```python
from build123d import *

# Parameters (mm, degrees)
EXTRU_MINCE1_DEPTH         = 2.3
CONG_1_R                   = 2.3
ESQUISSE2_W                = 40
ESQUISSE2_H                = 49.6
BOSS_EXTRU_1_DEPTH         = 2.3
R_P_TITION_LIN_AIRE1_COUNT = 2
R_P_TITION_LIN_AIRE1_PITCH = 40
CONG_2_R                   = 2.3
BOSS_EXTRU_2_DEPTH         = 40
ENL_V_START                = 37.8
ESQUISSE4_W                = 30
ESQUISSE4_H                = 12
ENL_V_MAT_EXTRU_1_DEPTH    = 35.5


with BuildPart() as part:
    # Esquisse1 → Extru.-Mince1 (new, symmetric)
    with BuildSketch(Plane.XY):
        Polygon((-4.3, -57), (-4.3, -47.3), (2.3, -47.3), (2.3, 2.3), (-8.9, 2.3), (-8.9, -12), (-4.3, -12), (-4.3, -2.3), (-2.3, -2.3), (-2.3, -42.7), (-8.9, -42.7), (-8.9, -57), align=None)
    extru_mince1 = extrude(amount=EXTRU_MINCE1_DEPTH, both=True)

    # Congé1
    cong_1_edges = [part.edges().sort_by_distance(p)[0] for p in [
        (-6.6, -57, -2.3),
        (-4.3, -52.15, -2.3),
        (-1, -47.3, -2.3),
        (2.3, -22.5, -2.3),
        (-3.3, 2.3, -2.3),
        (-8.9, -4.85, -2.3),
        (-6.6, -12, -2.3),
        (-4.3, -7.15, -2.3),
        (-3.3, -2.3, -2.3),
        (-2.3, -22.5, -2.3),
        (-5.6, -42.7, -2.3),
        (-8.9, -49.85, -2.3),
        (-5.6, -42.7, 2.3),
        (-2.3, -22.5, 2.3),
        (-3.3, -2.3, 2.3),
        (-4.3, -7.15, 2.3),
        (-6.6, -12, 2.3),
        (-8.9, -4.85, 2.3),
        (-3.3, 2.3, 2.3),
        (2.3, -22.5, 2.3),
        (-1, -47.3, 2.3),
        (-4.3, -52.15, 2.3),
        (-6.6, -57, 2.3),
        (-8.9, -49.85, 2.3),
    ]]
    fillet(cong_1_edges, radius=CONG_1_R - 0.0001)  # a hair under: the kernel refuses the full size

    # Esquisse2 → Boss.-Extru.1 (add)
    with BuildSketch(Plane(origin=(0, 0, 0), x_dir=(0, 0, -1), z_dir=(1, 0, 0))):
        with Locations((-20, -22.5)):
            Rectangle(ESQUISSE2_W, ESQUISSE2_H)
    extrude(amount=BOSS_EXTRU_1_DEPTH)

    # Répétition linéaire1: Extru.-Mince1 ×2
    with Locations(*[(0, 0, i * R_P_TITION_LIN_AIRE1_PITCH) for i in range(1, R_P_TITION_LIN_AIRE1_COUNT)]):
        add(extru_mince1)

    # Congé2
    cong_2_edges = [part.edges().sort_by_distance(p)[0] for p in [
        (-5.6, -42.7, 42.3),
        (-2.3, -22.5, 42.3),
        (-3.3, -2.3, 42.3),
        (-4.3, -7.15, 42.3),
        (-6.6, -12, 42.3),
        (-8.9, -4.85, 42.3),
        (-3.3, 2.3, 42.3),
        (2.3, -22.5, 42.3),
        (-6.6, -57, 42.3),
        (-4.3, -52.15, 42.3),
        (-1, -47.3, 42.3),
        (-8.9, -49.85, 42.3),
        (-2.15, -47.3, 37.7),
        (-4.3, -52.15, 37.7),
        (-6.6, -57, 37.7),
        (-8.9, -49.85, 37.7),
        (-5.6, -42.7, 37.7),
        (-2.3, -22.5, 37.7),
        (-3.3, -2.3, 37.7),
        (-4.3, -7.15, 37.7),
        (-6.6, -12, 37.7),
        (-8.9, -4.85, 37.7),
        (-4.45, 2.3, 37.7),
    ]]
    fillet(cong_2_edges, radius=CONG_2_R - 0.0001)  # a hair under: the kernel refuses the full size

    # Esquisse3 → Boss.-Extru.2 (add)
    with BuildSketch(Plane.XY):
        with BuildLine():
            Line((2.3, -39.8), (2.3, -13.05))
            Line((2.3, -13.05), (4.894555434, -13.05))
            ThreePointArc((4.894555434, -13.05), (20.05, -21.8), (35.205444566, -13.05))
            Line((35.205444566, -13.05), (37.8, -13.05))
            ThreePointArc((37.8, -13.05), (33.502205526, -23.477720869), (23.084609691, -27.8))
            Line((23.084609691, -27.8), (2.3, -39.8))
        make_face()
    extrude(amount=BOSS_EXTRU_2_DEPTH)

    # Esquisse4 → Enlèv. mat.-Extru.1 (cut)
    with BuildSketch(Plane(origin=(0, 0, 0), x_dir=(0, 0, -1), z_dir=(1, 0, 0)).offset(ENL_V_START)):
        with Locations((-20, -33.8)):
            Rectangle(ESQUISSE4_W, ESQUISSE4_H)
    extrude(amount=-ENL_V_MAT_EXTRU_1_DEPTH, mode=Mode.SUBTRACT)


solid = part.part
```
Could you check a few things on this model? Use its own coordinates, in mm. A direction names the side the tool comes from. Round coordinates to 2 decimals unless told otherwise and drop trailing zeros. Loops run counter-clockwise (first coordinate to the right, second up) from the corner with the lowest first, then second, coordinate; pieces in that order, holes last. Notation, with made-up numbers: M -28.5,86.25 L 14.5,86.25 A16 cw 14.5,107.25 Z; hole C 69,63 d6. An arc over 180 degrees is marked long. Put each result on its own line as item: value.
Q1. Imagine slicing it at C-C (z = 31.5). Write out the boundary of the cut face in (x, y).
Check result:
outline: M 0,-47.3 L 2.3,-47.3 L 2.3,-27.8 L 23.08,-27.8 A14.72 ccw 37.8,-13.05 L 35.21,-13.05 A17.5 cw 4.89,-13.05 L 2.3,-13.05 L 2.3,2.3 L 0,2.3 Z
Q2. I need wall thicknesses on probe 1 along Y at (x, z) = (3, 14); probe 2 along X at (y, z) = (-45.5, 28); probe 3 along X at (y, z) = (-20, 11). Which ranges of each line are inside material? Lowest first, please.
Check result:
probe 1: -27.8 to -13.05
probe 2: 0 to 2.3
probe 3: 0 to 12.32, 27.78 to 36.07
Q3. On a 3-axis mill with a long thin cutter (end or side, diameter ignored), from which of +Z, -Z, +X, -X, +Y, -Y can I reach the whole of each face in a straight line? I mean faces 4 (the face through (-6.568, -56.598, 1.298)), 5 (the face through (-8.24, -4.95, 1.61)), 6 (the face through (2.3, -28, 20)), 7 (the face through (-4.96, -5.92, 38.39)), 8 (the face through (-4.96, -5.92, 41.61)). Say none if no direction works.
Check result:
face 4: +X, -X, -Y
face 5: -X, +Y, -Y
face 6: +X
face 7: none
face 8: +Z
Q4. Thinking about a two-plate mould opening in Y: for faces 1 (the face through (1, 2.3, 20)), 2 (the face through (-4.96, -50.92, 41.61)), 3 (the face through (-3.25, -1.34, -1.87)), which applies, released by +Y, released by -Y, zero draft, split by the parting line, or undercut?
Check result:
face 1: released by +Y
face 2: zero draft
face 3: undercut
Q5. For pin 1 (6 mm diameter, centred on y = -8.5, z = 4.5, fed in from -X); pin 2 (5 mm diameter, centred on y = -44, z = 16, fed in from -X); pin 3 (10.5 mm diameter, centred on x = 13.5, z = 15, fed in from -Y), each with a flat end and sliding along its axis, tell me the tip position at first contact or that it passes through.
Check result:
pin 1: x = -8.34
pin 2: x = 0
pin 3: y = -27.8
Q6. Imagine slicing it at A-A (y = -7). State how many separate pieces and enclosed holes the cut face has, then the cut area to 3 significant figures.
Check result:
separate pieces: 3
enclosed holes: 0
area: 150 mm2
